Verification items for the finished model (mm, model axes). Face numbers are marked on the shaded views. A direction names the side the tool comes from. Coordinates: 2 decimals unless noted, no trailing zeros. Write each loop counter-clockwise with the first axis right and the second up, starting at its lowest first coordinate (ties: lowest second). Pieces come first, ordered by that corner, then holes. Notation, with made-up numbers: (38.5, 47.25) -> (73.5, 47.25) arc R20 cw to (73.5, 60.25) -> close; hole circle Ø5 at (-14.75, 57.5). An arc over 180 degrees is marked (long way). Answer in a Markdown table with one row per item.
```python
from build123d import *

# Parameters (mm, degrees)
SKETCH1_W           = 20
SKETCH1_H           = 2
BOSS_EXTRUDE1_DEPTH = 30
SKETCH2_W           = 40
SKETCH2_H           = 40
BOSS_EXTRUDE2_DEPTH = 20
FILLET1_R           = 10


with BuildPart() as part:
    # Sketch1 → Boss-Extrude1 (new body)
    with BuildSketch(Plane.XY):
        with Locations((-20, -1)):
            Rectangle(SKETCH1_W, SKETCH1_H)
    extrude(amount=BOSS_EXTRUDE1_DEPTH)

    # Sketch2 → Boss-Extrude2 (add)
    with BuildSketch(Plane.XY):
        with Locations((-10, 18)):
            Rectangle(SKETCH2_W, SKETCH2_H)
    extrude(amount=-BOSS_EXTRUDE2_DEPTH)

    # Fillet1
    # the kernel refuses this fillet: 10 mm, written as the material it adds along each edge
    with BuildSketch(Plane(origin=(-10, 0, 0), x_dir=(0, 1, 0), z_dir=(-1, 0, 0))) as fillet1_piece_1:
        with BuildLine():
            CenterArc((FILLET1_R, -FILLET1_R), FILLET1_R, 90, 90)
            Line((0, -FILLET1_R), (0, 0))
            Line((0, 0), (FILLET1_R, 0))
        make_face()
    extrude(amount=20)
    # the kernel refuses this fillet: 10 mm, written as the material it takes off along each edge
    with BuildSketch(Plane(origin=(10, 38, 25), x_dir=(-1, 0, 0), z_dir=(0, 0, -1))) as fillet1_2_piece_1:
        with BuildLine():
            CenterArc((FILLET1_R, -FILLET1_R), FILLET1_R, 90, 90)
            Line((0, -FILLET1_R), (0, 0))
            Line((0, 0), (FILLET1_R, 0))
        make_face()
    extrude(amount=70, mode=Mode.SUBTRACT)
    with BuildSketch(Plane(origin=(5, 0, 30), x_dir=(0, 0, -1), z_dir=(-1, 0, 0))) as fillet1_2_piece_2:
        with BuildLine():
            CenterArc((6, 10), FILLET1_R, 233.130102354, 36.869897646)
            Line((0, 2), (0, 0))
            Line((0, 0), (6, 0))
        make_face()
    extrude(amount=50, mode=Mode.SUBTRACT)


solid = part.part
```
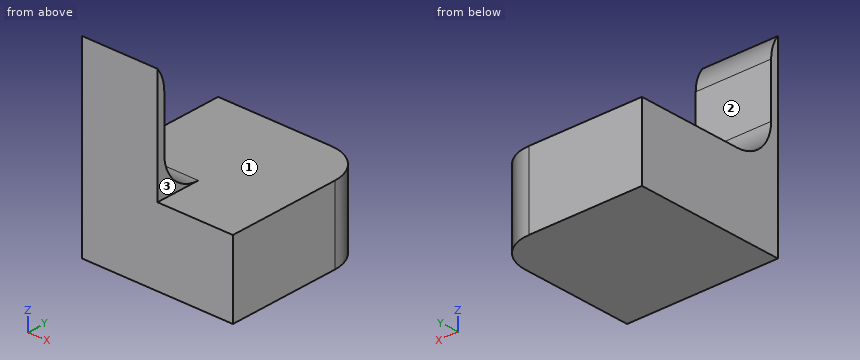
1. Section check D-D, the plane x = -4.5. Record the boundary of the cut face in (y, z).
Geometry says:
| item | result |
|---|---|
| outline | (-2, -20) -> (38, -20) -> (38, 0) -> (-2, 0) -> close |
2. Tool access check on the marked faces 1, 2 and 3. Record the directions out of +Z, -Z, +X, -X, +Y, -Y that give a thin tool (end or side, any length) a straight path to the whole face; none if there is none.
Geometry says:
| item | result |
|---|---|
| face 1 | +Z, +X, +Y |
| face 2 | +Z, +X, -X, +Y |
| face 3 | +Z, +X, +Y, -Y |
3. Depth check by flat-ended pin: P1, Ø11, axis at x = -21.5, z = 18, coming from the +Y side; P2, Ø5, axis at x = -20, y = 30.5, coming from the +Z side. Enter the tip coordinate at first touch or a pass-through.
Geometry says:
| item | result |
|---|---|
| P1 | y = 0 |
| P2 | z = 0 |
4. Section check A-A, the plane x = -21. Record the boundary of the cut face in (y, z).
Geometry says:
| item | result |
|---|---|
| outline | (-2, -20) -> (38, -20) -> (38, 0) -> (10, 0) arc R10 cw to (0, 10) -> (0, 24) arc R10 ccw to (-2, 30) -> close |
5. Section check C-C, the plane y = 8. Record the boundary of the cut face in (x, z), plus the area to 3 significant figures.
Geometry says:
| item | result |
|---|---|
| outline | (-30, -20) -> (10, -20) -> (10, 0) -> (-10, 0) -> (-10, 0.2) -> (-30, 0.2) -> close |
| area | 804 mm^2 |
6. Thickness scan on line 1 (Z direction, x = -21, y = 22); line 2 (Y direction, x = -14.5, z = 17); line 3 (Y direction, x = -18, z = 3.5). Record the ranges inside material, lowest first. Write a range as from..to.
Geometry says:
| item | result |
|---|---|
| line 1 | -20..0 |
| line 2 | -2..0 |
| line 3 | -2..2.4 |
7. Section check B-B, the plane z = 17.5. Record the boundary of the cut face in (x, y).
Geometry says:
| item | result |
|---|---|
| outline | (-30, -2) -> (-10, -2) -> (-10, 0) -> (-30, 0) -> close |
